Geometry: final body of the model. Coordinates: model frame, mm. Coordinates: 2 decimals unless noted, no trailing zeros. Loops run counter-clockwise (first coordinate to the right, second up) from the corner with the lowest first, then second, coordinate; pieces in that order, holes last. Notation, with made-up numbers: (-18, 58) - (23, 58) arc R12 ccw to (23, 78) - close; hole circle Ø7 at (-19, 26). An arc over 180 degrees is marked (long way). Put each result on its own line as item: value. Start each with the question number.
1) Material intervals for line 1 along Y through (x, z) = (5, 6.75); line 2 along X through (y, z) = (56, 8.5); line 3 along X through (y, z) = (3, 0.5), sorted ascending. Write a range as from..to.
2) Contact query for a flat-ended pin moving along its axis: pin 1 Ø6.5 at (x, y) = (50, 55) entering from +Z. Output: stop coordinate, or through.
3) Section B-B on y = 5. Output: boundary loops of the cut face in (x, z), and give its area (3 significant figures).
4) Draft query along Y for faces 1 (the cylindrical face through (7.385, 5.751, 4.93)), 2 (the flat face through (-10, 29, 5)), 3 (the flat face through (27, 70, 5)). Return one class per face: +Y half, -Y half, draft (parallel to the pull), parting line (faces both ways), or undercut.
5) Section A-A on x = 5. Output: boundary loops of the cut face in (y, z), and give its area (3 significant figures).
```python
from build123d import *

# Parameters (mm, degrees)
SKETCH1_W           = 75
SKETCH1_H           = 80
SKETCH1_W_2         = 55
SKETCH1_H_2         = 60
SKETCH1_R           = 2.5
BOSS_EXTRUDE1_DEPTH = 10


with BuildPart() as part:
    # Sketch1 → Boss-Extrude1 (new body)
    with BuildSketch(Plane.XY):
        with Locations((27.5, 30)):
            Rectangle(SKETCH1_W, SKETCH1_H)
        with Locations((27.5, 30)):
            Rectangle(SKETCH1_W_2, SKETCH1_H_2, mode=Mode.SUBTRACT)
        with Locations((27.5, 30)):
            Rectangle(SKETCH1_W_2, SKETCH1_H_2)
        with Locations((50, 5)):
            Circle(SKETCH1_R, mode=Mode.SUBTRACT)
        with Locations((5, 5)):
            Circle(SKETCH1_R, mode=Mode.SUBTRACT)
        with Locations((5, 55)):
            Circle(SKETCH1_R, mode=Mode.SUBTRACT)
        with Locations((50, 55)):
            Circle(SKETCH1_R, mode=Mode.SUBTRACT)
    extrude(amount=BOSS_EXTRUDE1_DEPTH)


solid = part.part
```
Answer block:
1. line 1: y = -10..2.5, 7.5..52.5, 57.5..70
1. line 2: x = -10..2.71, 7.29..47.71, 52.29..65
1. line 3: x = -10..3.5, 6.5..48.5, 51.5..65
2. pin 1: stops at z = 10
3. outline: (-10, 0) - (2.5, 0) - (2.5, 10) - (-10, 10) - close; (7.5, 0) - (47.5, 0) - (47.5, 10) - (7.5, 10) - close; (52.5, 0) - (65, 0) - (65, 10) - (52.5, 10) - close
3. area: 650 mm²
4. face 1: undercut
4. face 2: draft
4. face 3: +Y half
5. outline: (-10, 0) - (2.5, 0) - (2.5, 10) - (-10, 10) - close; (7.5, 0) - (52.5, 0) - (52.5, 10) - (7.5, 10) - close; (57.5, 0) - (70, 0) - (70, 10) - (57.5, 10) - close
5. area: 700 mm²
